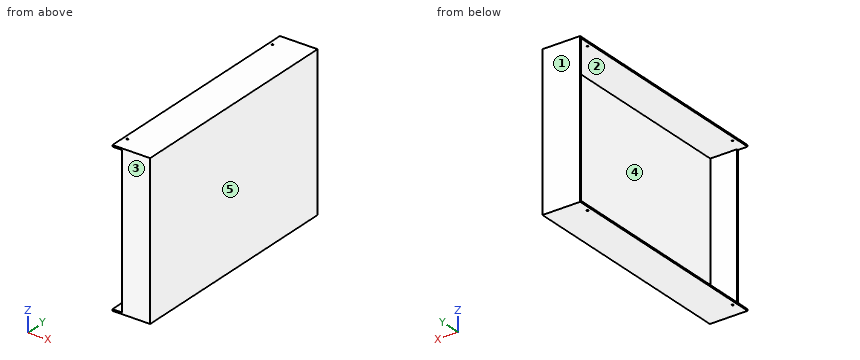
Autodesk Inventor part; units mm, degrees
ref_plane "YZ Plane" through (0, 0, 0) normal (1, 0, 0) x (0, 1, 0)
ref_plane "XZ Plane" through (0, 0, 0) normal (0, 1, 0) x (-1, 0, 0)
ref_plane "XY Plane" through (0, 0, 0) normal (0, 0, 1) x (1, 0, 0)
sketch "Эскиз1" plane through (0, 0, 0) normal (1, 0, 0) x (0, 1, 0)
  line L0 (-300, 200) -> (300, 200)
  line L1 (300, 200) -> (300, -200)
  line L2 (300, -200) -> (-300, -200)
  line L3 (-300, -200) -> (-300, 200)
  line L4 (-300, 200) -> (300, -200) construction
  line L5 (300, 200) -> (-300, -200) construction
  point P0 (0, 0)
  dimension "d0" = 400
  dimension "d1" = 600
extrude "Выдавливание1" add sketch "Эскиз1" along normal blind 4
sketch "Эскиз2" plane through (0, 0, 0) normal (-1, 0, 0) x (0, 0, 1)
  line L0 (-200, -300) -> (-200, 300)
  line L1 (-200, 300) -> (200, 300)
  line L2 (-200, -300) -> (-196, -300)
  line L3 (-196, -300) -> (-196, 300)
  line L4 (-196, 300) -> (-200, 300)
  line L5 (-200, 300) -> (-200, -300)
  line L6 (200, 300) -> (200, -300)
  line L7 (-200, 300) -> (200, 300)
  line L8 (200, 300) -> (200, 296)
  line L9 (200, 296) -> (-200, 296)
  line L10 (-200, 296) -> (-200, 300)
  line L11 (200, -300) -> (196, -300)
  line L12 (196, -300) -> (196, 300)
  line L13 (196, 300) -> (200, 300)
  line L14 (200, 300) -> (200, -300)
  point P0 (0, 0)
  point P1 (-196, 296)
  point P2 (196, 296)
  dimension "d4" = 4
  dimension "d5" = 4
  dimension "d6" = 4
extrude "Выдавливание2" add sketch "Эскиз2" along normal blind 95
sketch "Эскиз3" plane through (0, 0, 0) normal (-1, 0, 0) x (0, 0, 1)
  line L0 (-200, 300) -> (-200, -300)
  line L1 (200, -300) -> (200, 300)
  line L2 (-200, -300) -> (200, -300)
  line L3 (200, -300) -> (200, -296)
  line L4 (200, -296) -> (-200, -296)
  line L5 (-200, -296) -> (-200, -300)
  point P0 (0, 0)
  point P1 (-200, -296)
  dimension "d10" = 4
extrude "Выдавливание3" add sketch "Эскиз3" along normal blind 70
sketch "Эскиз4" plane through (4, -300, -200) normal (0, 0, -1) x (-1, 0, 0)
  line L0 (4, 300) -> (99, 300) construction
  line L1 (99, 0) -> (99, 600)
  line L2 (0, 0) -> (99, 0)
  point P0 (89, 560)
  point P1 (89, 40)
  dimension "d13" = 10
  dimension "d14" = 40
hole "Отверстие1" at (-85, 260, -200) at (-85, -260, -200) direction (0, 0, 1) diameter 3.9 depth 6 countersink diameter 4.5 countersink angle 90
sketch "Эскиз5" plane through (4, -300, 200) normal (0, 0, 1) x (1, 0, 0)
  circle A0 centre (-89, 560) radius 2.25
  circle A1 centre (-89, 40) radius 2.25
  point P0 (-4, 300)
hole "Отверстие2" at (-85, 260, 200) at (-85, -260, 200) direction (0, 0, -1) diameter 3.9 depth 6 countersink diameter 4 countersink angle 90
equation "\"d5\" = d4"
equation "\"d6\" = d4"
properties part number "Стеклянная крышка"
Build history of the part. All positions in model axes, mm. Face numbers are marked on the shaded views. A direction names the side the tool comes from. Round coordinates to 2 decimals unless told otherwise and drop trailing zeros. Write each loop counter-clockwise with the first axis right and the second up, starting at its lowest first coordinate (ties: lowest second). Pieces come first, ordered by that corner, then holes. Notation, with made-up numbers: (-34.5, 1.25) - (-30.5, 1.25) arc R25 ccw to (-30.5, 30.25) - close; hole circle Ø2 at (52.5, -23.75). An arc over 180 degrees is marked (long way). Use CSV: the item, a comma, the result in double quotes.
(1) Band-saw the part on B-B (z = -84). Write the cut outline in (x, y).
Response:
outline,"(-95, 296) - (0, 296) - (0, -296) - (-70, -296) - (-70, -300) - (4, -300) - (4, 300) - (-95, 300) - close"
(2) Wall check: line 1 (Y direction, x = -85, z = 197); line 2 (Z direction, x = -55, y = 97.5); line 3 (X direction, y = 260, z = 197.4). Give the ranges that are in metal, low to high.
Response:
line 1,"-300 to -261.95, -258.05 to 258.05, 261.95 to 300"
line 2,"-200 to -196, 196 to 200"
line 3,"-95 to -86.95, -83.05 to 4"
(3) Pin check, flat tips, straight feed: P1, Ø6, axis at x = -85, y = -260, coming from the +Z side; P2, Ø4, axis at y = 111.5, z = 141.5, coming from the -X side; P3, Ø1.2, axis at y = -299, z = -75.5, coming from the -X side. Stop position of each tip, or through.
Response:
P1,"z = 200"
P2,"x = 0"
P3,"x = -70"
(4) Band-saw the part on C-C (x = -43.5). Write the cut outline in (y, z).
Response:
outline,"(-300, -200) - (300, -200) - (300, 200) - (-300, 200) - close; hole (-296, -196) - (296, -196) - (296, 196) - (-296, 196) - close"
(5) 3-axis set-ups, long thin cutter, end or side, ignore diameter. For the marked faces 1 and 2: which of +Z, -Z, +X, -X, +Y, -Y reach the whole face in a straight line?
Response:
face 1,"+Z, -Z, +X, -X, +Y"
face 2,"-X"
(6) Mould opens along Y. For the marked faces 3, 4 and 5 say: pulls with the +Y half, pulls with the -Y half, needs draft (parallel to the pull), parting line crosses it, or undercut.
Response:
face 3,"pulls with the -Y half"
face 4,"undercut"
face 5,"needs draft"
(7) Band-saw the part on A-A (y = -123.5). Write the cut outline in (x, z), plus the area to 3 significant figures.
Response:
outline,"(-95, -200) - (4, -200) - (4, 200) - (-95, 200) - (-95, 196) - (0, 196) - (0, -196) - (-95, -196) - close"
area,"2,360 mm²"
